from build123d import *

# Parameters (mm, degrees)
BOSS_EXTRUDE1_DEPTH         = 10
M4_TAPPED_HOLE1_D           = 3.3
M4_TAPPED_HOLE1_DEPTH       = 10.1
M4_TAPPED_HOLE1_CSINK_D     = 4.05
M4_TAPPED_HOLE1_CSINK_ANGLE = 90
M4_TAPPED_HOLE1_TIP         = 0.991420021
FILLET1_R                   = 8
CHAMFER1_SIZE               = 1
SKETCH4_R                   = 1
CUT_EXTRUDE1_DEPTH          = 10
SKETCH6_W                   = 3.5
SKETCH6_H                   = 16
CUT_EXTRUDE3_DEPTH          = 4
FILLET3_R                   = 2


with BuildPart() as part:
    # Sketch1 → Boss-Extrude1 (new body)
    with BuildSketch(Plane.XY):
        Polygon((-50, 8), (50, 8), (50, -8), (-50, -8), (-50, -5), (-46, -5), (-46, 5), (-50, 5), align=None)
    extrude(amount=BOSS_EXTRUDE1_DEPTH)

    # M4 Tapped Hole1
    with Locations(Plane(origin=(-46, 0, 5), x_dir=(0, 0, -1), z_dir=(-1, 0, 0))):
        with Locations((0, 0)):
            CounterSinkHole(M4_TAPPED_HOLE1_D / 2, M4_TAPPED_HOLE1_CSINK_D / 2, depth=M4_TAPPED_HOLE1_DEPTH, counter_sink_angle=M4_TAPPED_HOLE1_CSINK_ANGLE)
            with Locations((0, 0, -(M4_TAPPED_HOLE1_DEPTH + M4_TAPPED_HOLE1_TIP / 2))):  # 118° drill point
                Cone(0, M4_TAPPED_HOLE1_D / 2, M4_TAPPED_HOLE1_TIP, mode=Mode.SUBTRACT)

    # Fillet1
    fillet1_edges = [part.edges().sort_by_distance(p)[0] for p in [
        (50, 8, 5),
        (50, -8, 5),
    ]]
    fillet(fillet1_edges, radius=FILLET1_R - 0.0001)  # a hair under: the kernel refuses the full size

    # Chamfer1
    chamfer1_edges = [part.edges().sort_by_distance(p)[0] for p in [
        (-3.99995, -8, 10),
        (-3.99995, 8, 0),
        (-3.99995, 8, 10),
        (47.656883539, -5.656883539, 0),
        (47.656883539, 5.656883539, 0),
        (47.656883539, -5.656883539, 10),
        (47.656883539, 5.656883539, 10),
        (-3.99995, -8, 0),
    ]]
    chamfer(chamfer1_edges, length=CHAMFER1_SIZE)

    # Sketch4 → Cut-Extrude1 (cut)
    with BuildSketch(Plane(origin=(0, 0, 0), x_dir=(-1, 0, 0), z_dir=(0, 0, -1))):
        with Locations((-42, 0)):
            Circle(SKETCH4_R)
        with Locations((-34, 0)):
            Circle(SKETCH4_R)
        with Locations((-26, 0)):
            Circle(SKETCH4_R)
        with Locations((-18, 0)):
            Circle(SKETCH4_R)
        with Locations((-10, 0)):
            Circle(SKETCH4_R)
        with Locations((-2, 0)):
            Circle(SKETCH4_R)
        with Locations((6, 0)):
            Circle(SKETCH4_R)
        with Locations((14, 0)):
            Circle(SKETCH4_R)
        with Locations((22, 0)):
            Circle(SKETCH4_R)
        with Locations((30, 0)):
            Circle(SKETCH4_R)
    extrude(amount=-CUT_EXTRUDE1_DEPTH, mode=Mode.SUBTRACT)

    # Sketch6 → Cut-Extrude3 (cut)
    with BuildSketch(Plane.ZY.offset(50)):
        with Locations((1.75, 0)):
            Rectangle(SKETCH6_W, SKETCH6_H)
    extrude(amount=-CUT_EXTRUDE3_DEPTH, mode=Mode.SUBTRACT)

    # Fillet3
    fillet3_edges = [part.edges().sort_by_distance(p)[0] for p in [
        (-48, 5, 3.5),
        (-48, -5, 3.5),
    ]]
    fillet(fillet3_edges, radius=FILLET3_R)


solid = part.part
Work out the finished part from the listing and answer in its coordinate system (mm). A direction names the side the tool comes from. Round coordinates to 2 decimals unless told otherwise and drop trailing zeros. Write each loop counter-clockwise with the first axis right and the second up, starting at its lowest first coordinate (ties: lowest second). Pieces come first, ordered by that corner, then holes. Notation, with made-up numbers: (55, -23) -> (88, -23) arc R21 cw to (88, -12) -> close; hole circle Ø6 at (-12, -30.75). An arc over 180 degrees is marked (long way). Answer as CSV lines item,"result". Start each with the question number.
(1) Each of these flat-tipped pins is pushed along its axis until it touches: pin 1 (0.8 mm diameter, centred on x = -48, y = 7.5, fed in from -Z); pin 2 (1.5 mm diameter, centred on y = 5.5, z = 3, fed in from +X). Where does it stop, or does it pass through?
(2) Find the intervals of material crossed by probe 1 along Y at (x, z) = (34, 5.25); probe 2 along Y at (x, z) = (-38, 6.25); probe 3 along X at (y, z) = (-1.75, 3.5), in increasing order.
(3) A tool of negligible diameter and unlimited length cuts with its end or side. For faces 5 (the flat face through (-46, 0.1, 2.7)), 6 (the flat face through (-48, 5, 8)), 7 (the flat face through (0, 0, 10)), from which of +Z, -Z, +X, -X, +Y, -Y can it reach the whole face along a straight path? Write none if from no direction.
(4) The mould has two halves that part along X. Classify faces 1 (the flat face through (-50, 6, 7)), 2 (the cylindrical face through (-5.2, -0.6, 4.9)), 3 (the cylindrical face through (-48.03, 5.57, 4.1)), 4 (the conical face through (47.118, -5.007, 0.16)): +X half, -X half, draft (parallel to the pull), parting line (faces both ways), or undercut.
(5) The part is cut by section A-A, the plane x = -14. Give the vertices of the cut face in (y, z).
Output values:
1,pin 1,"stops at z = 3.5"
1,pin 2,"stops at x = 48.44"
2,probe 1,"y = -8 to -1, 1 to 8"
2,probe 2,"y = -8 to -1.08, 1.08 to 8"
2,probe 3,"x = -46 to 49.81"
3,face 5,"-Z, -X"
3,face 6,"+Z, -Z, -X"
3,face 7,"+Z, +X, -X, +Y, -Y"
4,face 1,"-X half"
4,face 2,"undercut"
4,face 3,"draft"
4,face 4,"+X half"
5,outline,"(-8, 1) -> (-7, 0) -> (-1, 0) -> (-1, 10) -> (-7, 10) -> (-8, 9) -> close; (1, 0) -> (7, 0) -> (8, 1) -> (8, 9) -> (7, 10) -> (1, 10) -> close"
